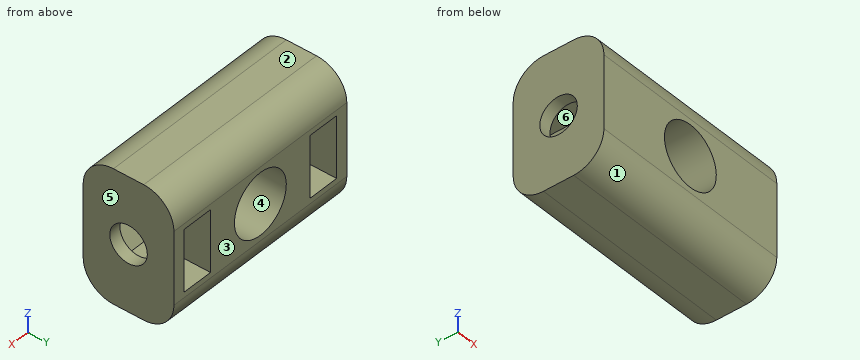
from build123d import *

# Parameters (mm, degrees)
CROQUIS1_W              = 34
CROQUIS1_H              = 22
CROQUIS1_R              = 5.1
SALIENTE_EXTRUIR1_DEPTH = 15
CORTAR_EXTRUIR1_DEPTH   = 5.2
CORTAR_EXTRUIR2_DEPTH   = 5.2
CROQUIS5_R              = 3.1
CORTAR_EXTRUIR4_DEPTH   = 4
CORTAR_EXTRUIR5_START   = -4
CROQUIS6_R              = 3.1
CORTAR_EXTRUIR5_DEPTH   = 4
REDONDEO1_R             = 5


with BuildPart() as part:
    # Croquis1 → Saliente-Extruir1 (new body)
    with BuildSketch(Plane(origin=(0, 0, 0), x_dir=(1, 0, 0), z_dir=(0, 1, 0))):
        with Locations((17, 11)):
            Rectangle(CROQUIS1_W, CROQUIS1_H)
        with Locations(Location((17, 11, 0), (0, 0, 270))):
            Circle(CROQUIS1_R, mode=Mode.SUBTRACT)
    extrude(amount=SALIENTE_EXTRUIR1_DEPTH)

    # Croquis2 → Cortar-Extruir1 (cut)
    with BuildSketch(Plane.ZY.offset(-2)):
        Polygon((-16.1, 10.444486373), (-16.1, 15), (-5.9, 15), (-5.9, 10.444486373), (-5.9, 4.555513627), (-11, 1.611027254), (-16.1, 4.555513627), align=None)
    extrude(amount=-CORTAR_EXTRUIR1_DEPTH, mode=Mode.SUBTRACT)

    # Croquis3 → Cortar-Extruir2 (cut)
    with BuildSketch(Plane(origin=(32, 0, 0), x_dir=(0, 0, -1), z_dir=(1, 0, 0))):
        Polygon((5.9, 15), (5.9, 4.555513627), (11, 1.611027254), (16.1, 4.555513627), (16.1, 15), align=None)
    extrude(amount=-CORTAR_EXTRUIR2_DEPTH, mode=Mode.SUBTRACT)

    # Croquis5 → Cortar-Extruir4 (cut)
    with BuildSketch(Plane(origin=(34, 0, 0), x_dir=(0, 0, -1), z_dir=(1, 0, 0))):
        with Locations((11, 7.5)):
            Circle(CROQUIS5_R)
    extrude(amount=-CORTAR_EXTRUIR4_DEPTH, mode=Mode.SUBTRACT)

    # Croquis6 → Cortar-Extruir5 (cut)
    with BuildSketch(Plane.ZY.offset(CORTAR_EXTRUIR5_START)):
        with Locations(Location((-11, 7.5, 0), (0, 0, 180))):
            Circle(CROQUIS6_R)
    extrude(amount=CORTAR_EXTRUIR5_DEPTH, mode=Mode.SUBTRACT)

    # Redondeo1
    redondeo1_edges = [part.edges().sort_by_distance(p)[0] for p in [
        (17, 15, -22),
        (17, 0, -22),
        (17, 0, 0),
        (17, 15, 0),
    ]]
    fillet(redondeo1_edges, radius=REDONDEO1_R)


solid = part.part
Input: part model. Units: mm. Frame: model coordinates. Face numbers are marked on the shaded views. A direction names the side the tool comes from. Round coordinates to 2 decimals unless told otherwise and drop trailing zeros. Loops run counter-clockwise (first coordinate to the right, second up) from the corner with the lowest first, then second, coordinate; pieces in that order, holes last. Notation, with made-up numbers: M 25,41 L 36,41 A20 ccw 36,64 Z; hole C 60,-4.75 d11. An arc over 180 degrees is marked long. Answer as CSV lines item,"result". Start each with the question number.
(1) Section D-D, the plane z = -7. Output: boundary loops of the cut face in (x, y), plus the area to 3 significant figures.
(2) Section B-B, the plane y = 7.5. Output: boundary loops of the cut face in (x, z), plus the area to 3 significant figures.
(3) Line query: line 1 (Z direction, x = 5.5, y = 10.25); line 2 (Z direction, x = 1.1, y = 7.5); line 3 (X direction, y = 8.5, z = -11). Output: solid intervals per line, ascending. Write a range as [from, to].
(4) First-contact query: pin 1 (1 mm diameter, centred on x = 12, z = -3, fed in from +Y); pin 2 (1 mm diameter, centred on x = 12.5, z = -19, fed in from -Y). Flat tips, straight axial feed; report the tip coordinate or a pass-through.
(5) Section C-C, the plane x = 24. Output: boundary loops of the cut face in (y, z).
(6) Draft query along Z for the marked faces 1, 2, 3 and 4. Return one class per face: released by +Z, released by -Z, zero draft, split by the parting line, or undercut.
(7) Section A-A, the plane x = 17. Output: boundary loops of the cut face in (y, z).
(8) Reachability of the marked faces 5 and 6 from +Z, -Z, +X, -X, +Y, -Y: full face, straight path, thin tool, end or side. Return the list, or none.
Values found:
1,outline,"M 0,0 L 13.84,0 L 13.84,15 L 7.2,15 L 7.2,3.92 L 2,3.92 L 2,15 L 0,15 Z; M 20.16,0 L 34,0 L 34,15 L 32,15 L 32,3.92 L 26.8,3.92 L 26.8,15 L 20.16,15 Z"
1,area,"300 mm²"
2,outline,"M 0,-22 L 34,-22 L 34,-14.1 L 32,-14.1 L 32,-16.1 L 26.8,-16.1 L 26.8,-5.9 L 32,-5.9 L 32,-7.9 L 34,-7.9 L 34,0 L 0,0 L 0,-7.9 L 2,-7.9 L 2,-5.9 L 7.2,-5.9 L 7.2,-16.1 L 2,-16.1 L 2,-14.1 L 0,-14.1 Z; hole C 17,-11 d10.2"
2,area,"535 mm²"
3,line 1,"z = [-21.99, -16.1], [-5.9, -0.01]"
3,line 2,"z = [-22, -14.1], [-7.9, 0]"
3,line 3,"x = [7.2, 11.9], [22.1, 26.8]"
4,pin 1,"stops at y = 14.77"
4,pin 2,"stops at y = 0.23"
5,outline,"M 0,-17 A5 ccw 5,-22 L 10,-22 A5 ccw 15,-17 L 15,-5 A5 ccw 10,0 L 5,0 A5 ccw 0,-5 Z"
6,face 1,"released by -Z"
6,face 2,"released by +Z"
6,face 3,"zero draft"
6,face 4,"undercut"
7,outline,"M 0,-17 A5 ccw 5,-22 L 10,-22 A5 ccw 15,-17 L 15,-16.1 L 0,-16.1 Z; M 0,-5.9 L 15,-5.9 L 15,-5 A5 ccw 10,0 L 5,0 A5 ccw 0,-5 Z"
8,face 5,"+Z, -Z, +X, +Y, -Y"
8,face 6,"+Y"
